```python
from build123d import *

# Parameters (mm, degrees)
BOSS_EXTRUDE1_DEPTH     = 4.4
CUT_EXTRUDE2_DEPTH      = 13.739679342
CUT_EXTRUDE2_DEPTH_BACK = 13.739679342


with BuildPart() as part:
    # Sketch1 → Boss-Extrude1 (new body)
    with BuildSketch(Plane.XY):
        with BuildLine():
            Line((-4, 3.769318743), (-3.5, -4.230681257))
            Line((-3.5, -4.230681257), (-5.5, -4.230681257))
            Line((-5.5, -4.230681257), (-6, 3.769318743))
            ThreePointArc((-6, 3.769318743), (-4.547652978, 8.455926386), (0, 10.297788342))
            ThreePointArc((0, 10.297788342), (4.547652978, 8.455926386), (6, 3.769318743))
            Line((6, 3.769318743), (5.5, -4.230681257))
            Line((5.5, -4.230681257), (3.5, -4.230681257))
            Line((3.5, -4.230681257), (4, 3.769318743))
            ThreePointArc((4, 3.769318743), (2.912733302, 6.839771433), (0, 8.297788342))
            ThreePointArc((0, 8.297788342), (-2.912733302, 6.839771433), (-4, 3.769318743))
        make_face()
    extrude(amount=BOSS_EXTRUDE1_DEPTH)

    # Sketch2 → Cut-Extrude2 (cut, two sides: drawn at the far end of the back side and taken through both)
    with BuildSketch(Plane.XY.offset(-CUT_EXTRUDE2_DEPTH_BACK)):
        Polygon((-3.5, -4.230681257), (-4.5, -4.230681257), (-3.590096666, -2.789134598), align=None)
        Polygon((3.5, -4.230681257), (3.590096666, -2.789134598), (4.5, -4.230681257), align=None)
    extrude(amount=CUT_EXTRUDE2_DEPTH + CUT_EXTRUDE2_DEPTH_BACK, mode=Mode.SUBTRACT)


solid = part.part
```
Can you work these out from the model? Positions are in its coordinate system, mm. A direction names the side the tool comes from. Round coordinates to 2 decimals unless told otherwise and drop trailing zeros. Loops run counter-clockwise (first coordinate to the right, second up) from the corner with the lowest first, then second, coordinate; pieces in that order, holes last. Notation, with made-up numbers: (-34, 9) -> (-24, 9) arc R13 cw to (-24, 24) -> close; hole circle Ø3 at (-23, -4.5). An arc over 180 degrees is marked (long way). One line per item, written item: value. Start each with the question number.
1. If we mould it in two halves opening along X, with no side actions, what happens to faces 4 (the flat face through (-5, -4.231, 2)), 5 (the cylindrical face through (2.943, 6.805, 2.169)), 6 (the flat face through (5.754, -0.175, 2.169)), 7 (the flat face through (4.04, -3.5, 2.17))? For each: pulls with the +X half, pulls with the -X half, needs draft (parallel to the pull), parting line crosses it, or undercut.
2. If I drill on probe 1 along X at (y, z) = (1.5, 4.15); probe 2 along X at (y, z) = (5, 0.3); probe 3 along Y at (x, z) = (-2.25, 2.15), over which ranges is the centre line in solid material (lowest first)?
3. If we section it at D-D, the plane x = -3: Write out the boundary of the cut face in (y, z), then the cut area to 3 significant figures.
4. For faces 1 (the flat face through (4.12, 3.14, 0)), 2 (the flat face through (-3.8, 0.54, 2.17)), 3 (the flat face through (-4.05, -3.52, 2.17)), which set-ups out of +Z, -Z, +X, -X, +Y, -Y let a thin tool reach every point of the face, with its end or its side?
5. If we section it at C-C, the plane z = 2.2: Write out the boundary of the cut face in (x, y).
6. For pin 1 (2 mm diameter, centred on x = -2, z = 3, fed in from -Y); pin 2 (5 mm diameter, centred on x = -4.5, y = 8, fed in from -Z); pin 3 (1.5 mm diameter, centred on x = 0.5, z = 1, fed in from -Y); pin 4 (1.5 mm diameter, centred on y = 8.5, z = 1.5, fed in from -X), each with a flat end and sliding along its axis, tell me the tip position at first contact or that it passes through.
7. If we section it at B-B, the plane x = 3.75: Write out the boundary of the cut face in (y, z).
8. If we section it at A-A, the plane y = 0: Write out the boundary of the cut face in (x, z).
Calculated:
1. face 4: needs draft
1. face 5: undercut
1. face 6: pulls with the +X half
1. face 7: undercut
2. probe 1: x = -5.86 to -3.86, 3.86 to 5.86
2. probe 2: x = -6.04 to -3.88, 3.88 to 6.04
2. probe 3: y = 7.45 to 9.98
3. outline: (6.74, 0) -> (9.65, 0) -> (9.65, 4.4) -> (6.74, 4.4) -> close
3. area: 12.8 mm²
4. face 1: -Z, +X, -X, +Y, -Y
4. face 2: +Z, -Z
4. face 3: +Z, -Z, -Y
5. outline: (-6, 3.77) -> (-5.5, -4.23) -> (-4.5, -4.23) -> (-3.59, -2.79) -> (-4, 3.77) arc R4.36 cw to (0, 8.3) arc R4.36 cw to (4, 3.77) -> (3.59, -2.79) -> (4.5, -4.23) -> (5.5, -4.23) -> (6, 3.77) arc R5.73 ccw to (0, 10.3) arc R5.73 ccw to start
6. pin 1: stops at y = 6.74
6. pin 2: stops at z = 0
6. pin 3: stops at y = 8.01
6. pin 4: stops at x = -5.1
7. outline: (-3.04, 0) -> (-0.23, 0) -> (-0.23, 4.4) -> (-3.04, 4.4) -> close; (5.42, 0) -> (9.18, 0) -> (9.18, 4.4) -> (5.42, 4.4) -> close
8. outline: (-5.76, 0) -> (-3.76, 0) -> (-3.76, 4.4) -> (-5.76, 4.4) -> close; (3.76, 0) -> (5.76, 0) -> (5.76, 4.4) -> (3.76, 4.4) -> close
